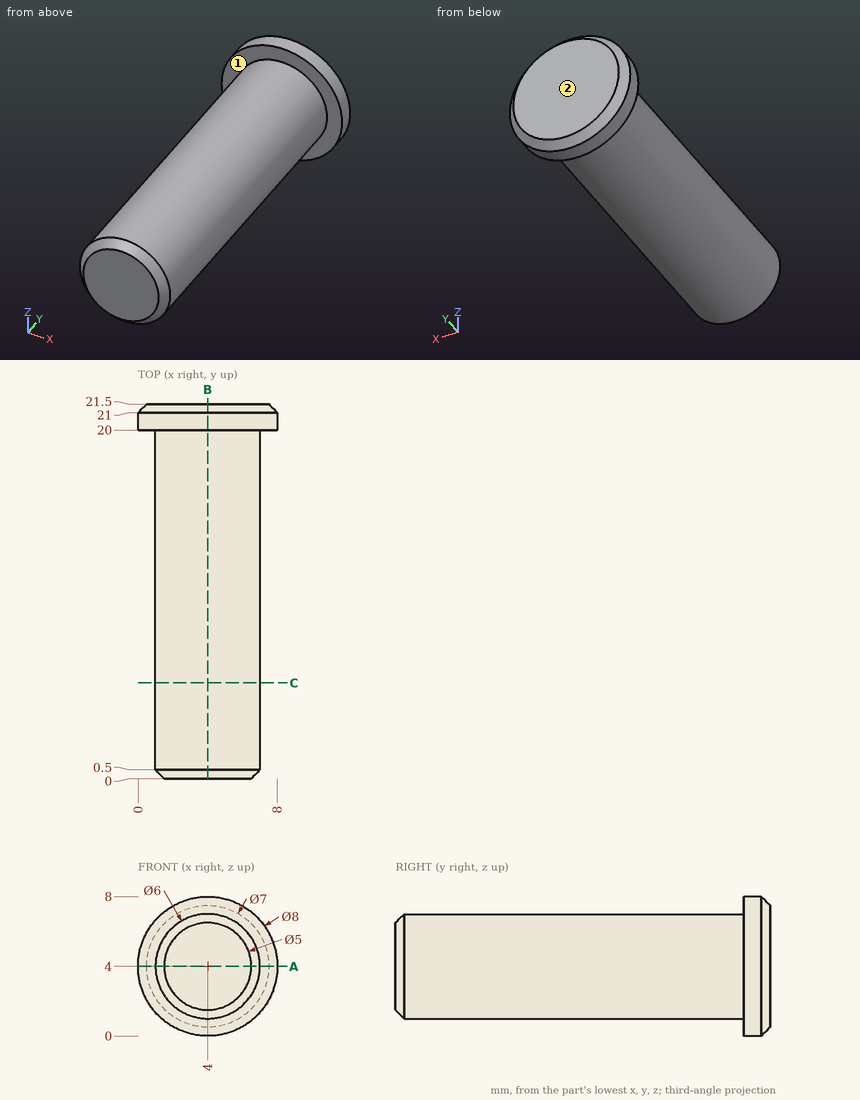
Geometry check sheet. Reference: drawing and pictorial views, mm from the part's lowest x, y, z. A direction names the side the tool comes from. Coordinates: 2 decimals unless noted, no trailing zeros. Order: outer loops, then holes, each group sorted by start corner. A loop starts at its lowest first (then second) coordinate and runs counter-clockwise, first axis right, second up.
Item 1: Section check C-C (y = 5.5). Enter the section's corners in (x, z), plus the area to 3 significant figures.
Item 2: Section check A-A (z = 4). Enter the section's corners in (x, y), plus the area to 4 significant figures.
Item 3: Depth check by flat-ended pin: pin 1 (4 mm diameter, centred on x = 6, z = 4.5, fed in from -Y); pin 2 (4 mm diameter, centred on y = 4.5, z = 7, fed in from -X). Enter the tip coordinate at first touch or a pass-through.
Item 4: Section check B-B (x = 4). Enter the section's corners in (y, z).
Item 5: Tool access check on the marked faces 1 and 2. Record the directions out of +Z, -Z, +X, -X, +Y, -Y that give a thin tool (end or side, any length) a straight path to the whole face; none if there is none.
Item 6: Scan lines: line 1 along Y through (x, z) = (3.5, 0.75); line 2 along Z through (x, y) = (4, 6.5); line 3 along Z through (x, y) = (1, 20.25). Record each from-to range of solid material in increasing order.
Check sheet entries:
1. outline: circle Ø6 at (4, 4)
1. area: 28.3 mm2
2. outline: (0, 20) - (1, 20) - (1, 0.5) - (1.5, 0) - (6.5, 0) - (7, 0.5) - (7, 20) - (8, 20) - (8, 21) - (7.5, 21.5) - (0.5, 21.5) - (0, 21) - close
2. area: 131.5 mm2
3. pin 1: stops at y = 0
3. pin 2: stops at x = 1.17
4. outline: (0, 1.5) - (0.5, 1) - (20, 1) - (20, 0) - (21, 0) - (21.5, 0.5) - (21.5, 7.5) - (21, 8) - (20, 8) - (20, 7) - (0.5, 7) - (0, 6.5) - close
5. face 1: -Y
5. face 2: +Z, -Z, +X, -X, +Y
6. line 1: y = 20 to 21.5
6. line 2: z = 1 to 7
6. line 3: z = 1.35 to 6.65
